```python
from build123d import *

# Parameters (mm, degrees)
BOSS_EXTRUDE1_DEPTH = 5
CHAMFER1_SIZE       = 3


with BuildPart() as part:
    # Sketch1 → Boss-Extrude1 (new, symmetric)
    with BuildSketch(Plane.XY):
        Polygon((20, 24), (11, 24), (11, 40), (0, 40), (0, 0), (20, 0), align=None)
    extrude(amount=BOSS_EXTRUDE1_DEPTH, both=True)

    # Chamfer1
    chamfer1_edges = [part.edges().sort_by_distance(p)[0] for p in [
        (10, 0, -5),
        (10, 0, 5),
    ]]
    chamfer(chamfer1_edges, length=CHAMFER1_SIZE)


solid = part.part
```
Part model, mm, in its own coordinate system. A direction names the side the tool comes from. Round coordinates to 2 decimals unless told otherwise and drop trailing zeros. Loops run counter-clockwise (first coordinate to the right, second up) from the corner with the lowest first, then second, coordinate; pieces in that order, holes last. Notation, with made-up numbers: (53, 53.25) -> (78, 53.25) arc R20 cw to (78, 90.25) -> close; hole circle Ø10 at (59, -38.5). An arc over 180 degrees is marked (long way). Use one line per item in the form item = value. Start each with the question number.
Item 1: Drop flat-ended pins along their axis: pin 1 Ø4.5 at (x, z) = (17.5, 1.5) entering from +Y; pin 2 Ø5 at (x, z) = (16, 3) entering from -Y. Give the stop position or say it passes through.
Item 2: Drill centre lines: line 1 along X through (y, z) = (28.5, 1.5); line 2 along Y through (x, z) = (10.5, -4); line 3 along Y through (x, z) = (12, -1.5). Where is each one in solid material? Low to high.
Item 3: Band-saw the part on C-C (y = 29). List the corners of the cut face in (x, z).
Item 4: Band-saw the part on B-B (x = 7.5). List the corners of the cut face in (y, z), plus the area to 3 significant figures.
Item 5: Tool access for faces 1 (the flat face through (16, 24, 0)), 2 (the flat face through (6, 40, 0)): list every direction of +Z, -Z, +X, -X, +Y, -Y with a clear straight run to the whole face (end or side of a thin tool).
Item 6: Band-saw the part on A-A (z = 3.5). List the corners of the cut face in (x, y), plus the area to 3 significant figures.
Data:
q1.pin_1 = 24
q1.pin_2 = 0
q2.line_1 = 0 to 11
q2.line_2 = 2 to 40
q2.line_3 = 0 to 24
q3.outline = (0, -5) -> (11, -5) -> (11, 5) -> (0, 5) -> close
q4.outline = (0, -2) -> (3, -5) -> (40, -5) -> (40, 5) -> (3, 5) -> (0, 2) -> close
q4.area = 391 mm^2
q5.face_1 = +Z, -Z, +X, +Y
q5.face_2 = +Z, -Z, +X, -X, +Y
q6.outline = (0, 1.5) -> (20, 1.5) -> (20, 24) -> (11, 24) -> (11, 40) -> (0, 40) -> close
q6.area = 626 mm^2
